The figure shows three views and two pictorial views of one solid part (mm, origin at its lowest corner). Answer the questions. A direction names the side the tool comes from. Coordinates: 2 decimals unless noted, no trailing zeros. Write each loop counter-clockwise with the first axis right and the second up, starting at its lowest first coordinate (ties: lowest second). Pieces come first, ordered by that corner, then holes. Notation, with made-up numbers: M 53,7.5 L 91,7.5 A18 ccw 91,12.5 Z; hole C -32.5,49.25 d9. An arc over 180 degrees is marked long. Write item = value, one per line. Start each with the question number.
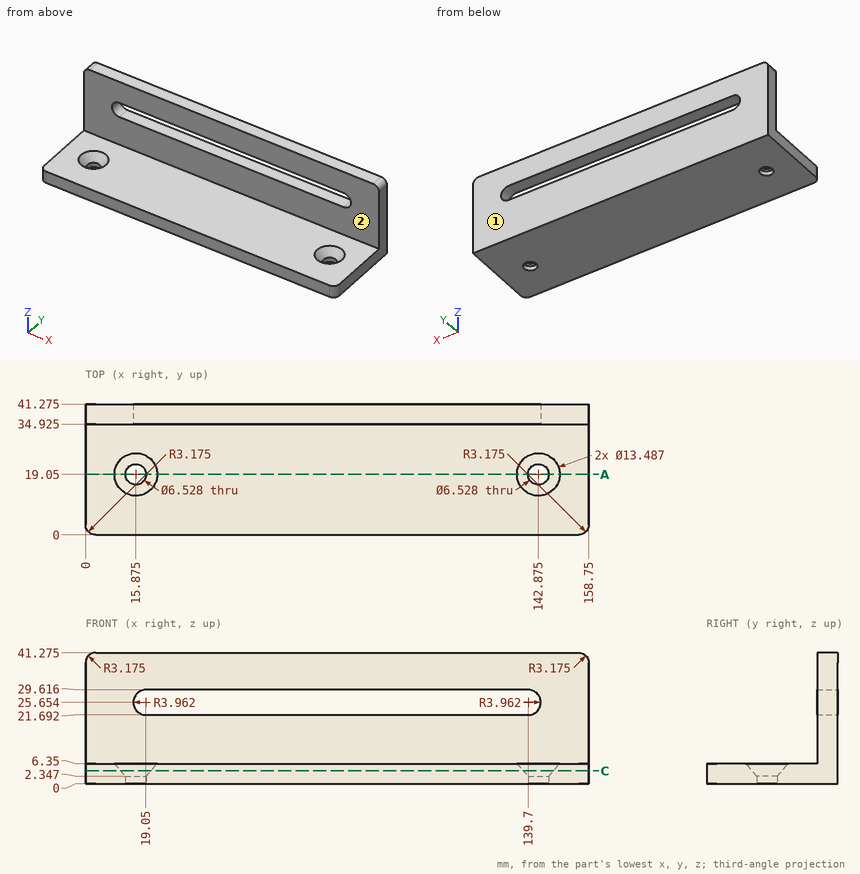
1. The part is cut by section A-A, the plane y = 19.05. Write down the section's boundary in (x, z).
2. Straight lines are drawn through the part: L1, parallel to X at y = 19.05, z = 1.55; L2, parallel to Y at x = 106.5, z = 19.5 (1 decimal); L3, parallel to Z at x = 21.5, y = 8. For each, find the intervals that lie inside material, in ascending order. Write a range as [from, to].
3. For the marked faces 1 and 2, determine the directions among +Z, -Z, +X, -X, +Y, -Y from which every point of the face is accessible in a straight line to the end or side of a thin tool.
4. Each of these flat-tipped pins is pushed along its axis until it touches: pin 1 (4 mm diameter, centred on x = 34.5, z = 28, fed in from -Y) (3 decimals); pin 2 (4 mm diameter, centred on x = 140, y = 6, fed in from +Z). Where does it stop, or does it pass through?
5. The part is cut by section C-C, the plane z = 4. Count the separate pieces of the cut face and the enclosed holes in it, and give its area (3 significant figures).
Solution:
q1.outline = M 0,0 L 12.61,0 L 12.61,2.35 L 9.13,6.35 L 0,6.35 Z; M 19.14,0 L 139.61,0 L 139.61,2.35 L 136.13,6.35 L 22.62,6.35 L 19.14,2.35 Z; M 146.14,0 L 158.75,0 L 158.75,6.35 L 149.62,6.35 L 146.14,2.35 Z
q2.L1 = [0, 12.61], [19.14, 139.61], [146.14, 158.75]
q2.L2 = [34.9, 41.3]
q2.L3 = [0, 6.35]
q3.face_1 = +Z, -Z, +X, -X, +Y
q3.face_2 = +Z, +X, -X, -Y
q4.pin_1 = 34.925
q4.pin_2 = 6.35
q5.separate_pieces = 1
q5.enclosed_holes = 2
q5.area = 6,410 mm^2
